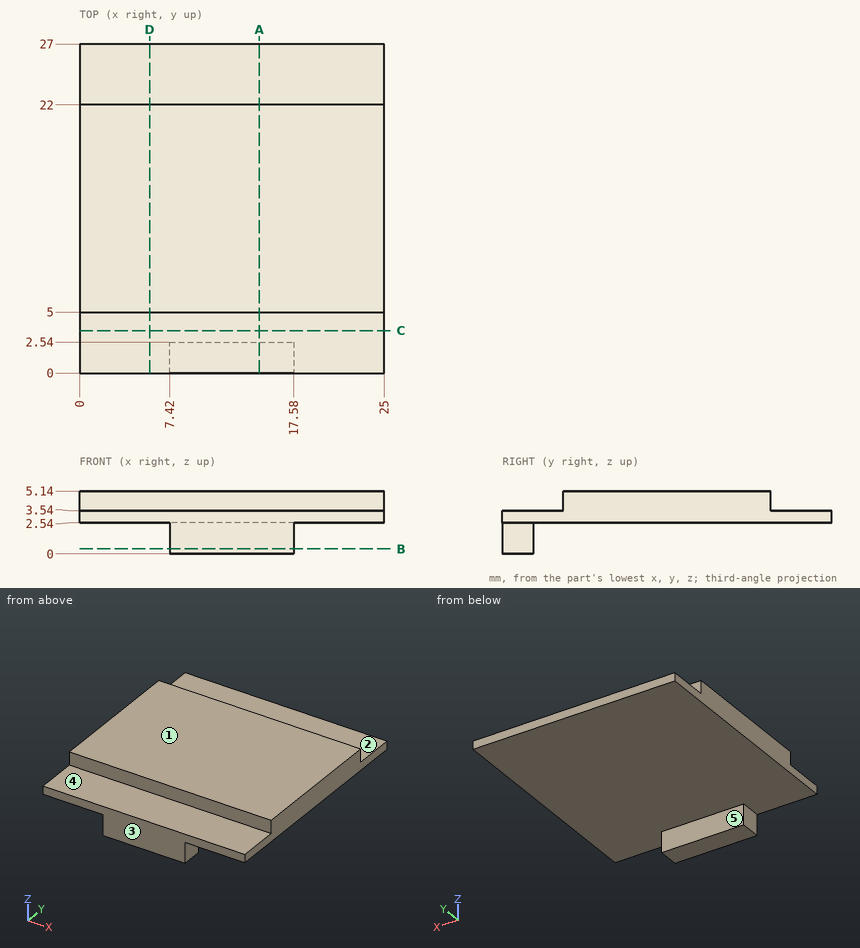
Geometry check sheet. Reference: drawing and pictorial views, mm from the part's lowest x, y, z. A direction names the side the tool comes from. Give positions to 0.01 mm unless a question says otherwise; leave off trailing zeros. Write each loop counter-clockwise with the first axis right and the second up, starting at its lowest first coordinate (ties: lowest second). Pieces come first, ordered by that corner, then holes. Notation, with made-up numbers: M 29,61 L 50,61 A23 cw 50,75 Z; hole C 30,12 d9. An arc over 180 degrees is marked long. Answer as CSV lines item,"result". Start each with the question number.
Q1. Section check C-C, the plane y = 3.5. Record the cut outline in (x, z), then the cut area to 3 significant figures.
Q2. Go/stop test with flat-tipped pins: pin 1 (0.8 mm diameter, centred on y = 1, z = 2, fed in from +X); pin 2 (2 mm diameter, centred on y = 1, z = 1.5, fed in from -X); pin 3 (4 mm diameter, centred on x = 8.5, y = 18.5, fed in from -Z); pin 4 (1.5 mm diameter, centred on x = 4, z = 1, fed in from +Y). Record where each tip stops, or that it passes through.
Q3. Material ranges on L1, parallel to Y at x = 10.5, z = 3.6; L2, parallel to Z at x = 8, y = 23.5; L3, parallel to Z at x = 5, y = 13, recorded low to high.
Q4. Tool access check on the marked faces 1, 2, 3, 4 and 5. Record the directions out of +Z, -Z, +X, -X, +Y, -Y that give a thin tool (end or side, any length) a straight path to the whole face; none if there is none.
Q5. Section check B-B, the plane z = 0.4. Record the cut outline in (x, y), then the cut area to 3 significant figures.
Q6. Section check A-A, the plane x = 14.75. Record the cut outline in (y, z).
Q7. Section check D-D, the plane x = 5.75. Record the cut outline in (y, z).
Geometry says:
1,outline,"M 0,2.54 L 25,2.54 L 25,3.54 L 0,3.54 Z"
1,area,"25.0 mm^2"
2,pin 1,"x = 17.58"
2,pin 2,"x = 7.42"
2,pin 3,"z = 2.54"
2,pin 4,"through"
3,L1,"5 to 22"
3,L2,"2.54 to 3.54"
3,L3,"2.54 to 5.14"
4,face 1,"+Z, +X, -X, +Y, -Y"
4,face 2,"+Z, +X, -X, +Y"
4,face 3,"+Z, -Z, +X, -X, -Y"
4,face 4,"+Z, +X, -X, -Y"
4,face 5,"-Z, +X, -X, +Y"
5,outline,"M 7.42,0 L 17.58,0 L 17.58,2.54 L 7.42,2.54 Z"
5,area,"25.8 mm^2"
6,outline,"M 0,0 L 2.54,0 L 2.54,2.54 L 27,2.54 L 27,3.54 L 22,3.54 L 22,5.14 L 5,5.14 L 5,3.54 L 0,3.54 Z"
7,outline,"M 0,2.54 L 27,2.54 L 27,3.54 L 22,3.54 L 22,5.14 L 5,5.14 L 5,3.54 L 0,3.54 Z"
